Check sheet for the modelled part. Datum: model origin and axes. Units: mm. Round coordinates to 2 decimals unless told otherwise and drop trailing zeros. Write each loop counter-clockwise with the first axis right and the second up, starting at its lowest first coordinate (ties: lowest second). Pieces come first, ordered by that corner, then holes. Notation, with made-up numbers: (5.25, -8) -> (25.25, -8) arc R32 ccw to (25.25, 20) -> close; hole circle Ø9 at (82, 87). An arc over 180 degrees is marked (long way). One line per item, written item: value.
from build123d import *

# Parameters (mm, degrees)
F0_W     = 55
F0_H     = 55
F1_DEPTH = 17.5
F3_DEPTH = 55.001
F5_DEPTH = 55.001


with BuildPart() as f1:
    # F0 (on Front) → F1 (new body, symmetric)
    with BuildSketch(Plane.XZ):
        Rectangle(F0_W, F0_H)
    extrude(amount=F1_DEPTH, both=True)

    # F2 (on face) → F3 (cut, through all)
    with BuildSketch(Plane.YZ.offset(27.5)):
        Polygon((-17.5, 27.5), (-17.5, -15.5), (17.5, 27.5), align=None)
    extrude(amount=-F3_DEPTH, mode=Mode.SUBTRACT)

    # F4 (on face) → F5 (cut, through all)
    with BuildSketch(Plane(origin=(0, 0, -27.5), x_dir=(1, 0, 0), z_dir=(0, 0, -1))):
        Polygon((8.5, 17.5), (27.5, -2.5), (27.5, 17.5), align=None)
    extrude(amount=-F5_DEPTH, mode=Mode.SUBTRACT)


solid = f1.part
Item 1: Depth check by flat-ended pin: pin 1 (1.5 mm diameter, centred on x = -7, y = -10.5, fed in from +Z); pin 2 (12 mm diameter, centred on x = -7, z = 8, fed in from -Y); pin 3 (5 mm diameter, centred on x = 19, z = -16, fed in from -Y). Enter the tip coordinate at first touch or a pass-through.
Result set:
pin 1: z = -5.98
pin 2: y = -3.26
pin 3: y = -9.08
Item 2: Sectioned sample at D-D (z = 0.5). Enter the section's corners in (x, y).
Result set:
outline: (-27.5, -4.48) -> (20.87, -4.48) -> (27.5, 2.5) -> (27.5, 17.5) -> (-27.5, 17.5) -> close
Item 3: Sectioned sample at B-B (x = 0). Enter the section's corners in (y, z), then the cut area to 3 significant figures.
Result set:
outline: (-17.5, -27.5) -> (17.5, -27.5) -> (17.5, 27.5) -> (-17.5, -15.5) -> close
area: 1,170 mm^2
Item 4: Material ranges on line 1 along Y through (x, z) = (8.5, 23.5); line 2 along Z through (x, y) = (6.5, 12.5); line 3 along X through (y, z) = (-1, -19) (3 decimals), recorded low to high.
Result set:
line 1: 14.24 to 17.5
line 2: -27.5 to 21.36
line 3: -27.5 to 24.175
Item 5: Sectioned sample at A-A (z = -7.5). Enter the section's corners in (x, y), then the cut area to 3 significant figures.
Result set:
outline: (-27.5, -10.99) -> (14.69, -10.99) -> (27.5, 2.5) -> (27.5, 17.5) -> (-27.5, 17.5) -> close
area: 1,480 mm^2
Item 6: Sectioned sample at C-C (y = -13). Enter the section's corners in (x, z) (3 decimals).
Result set:
outline: (-27.5, -27.5) -> (12.775, -27.5) -> (12.775, -9.971) -> (-27.5, -9.971) -> close
